Job drawing, mm, ordinate dimensions from the low corner. One solid piece. A direction names the side the tool comes from. Coordinates: 2 decimals unless noted, no trailing zeros. Write each loop counter-clockwise with the first axis right and the second up, starting at its lowest first coordinate (ties: lowest second). Pieces come first, ordered by that corner, then holes.
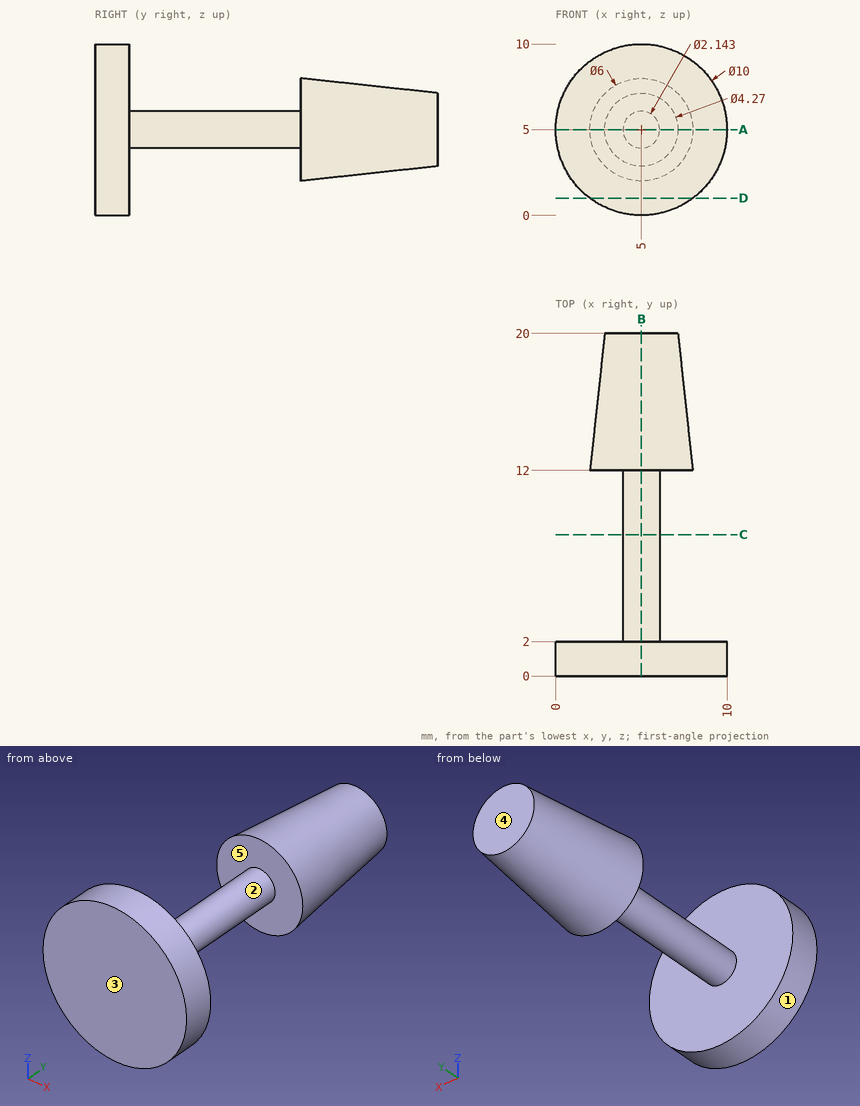
1. Saw through at C-C on y = 8.25. List the corners of the cut face in (x, z).
Computed values:
outline: circle Ø2.14 at (5, 5)
2. Saw through at A-A on z = 5. List the corners of the cut face in (x, y) (1 decimal).
Computed values:
outline: (0, 0) - (10, 0) - (10, 2) - (6.1, 2) - (6.1, 12) - (8, 12) - (7.1, 20) - (2.9, 20) - (2, 12) - (3.9, 12) - (3.9, 2) - (0, 2) - close
3. Saw through at B-B on x = 5. List the corners of the cut face in (y, z) (1 decimal).
Computed values:
outline: (0, 0) - (2, 0) - (2, 3.9) - (12, 3.9) - (12, 2) - (20, 2.9) - (20, 7.1) - (12, 8) - (12, 6.1) - (2, 6.1) - (2, 10) - (0, 10) - close
4. Flat gauge pins, fed straight in: pin 1 (6 mm diameter, centred on x = 3, y = 8.5, fed in from -Z); pin 2 (1.5 mm diameter, centred on x = 5.5, y = 16, fed in from +Z) (1 decimal); pin 3 (4 mm diameter, centred on x = 4.5, y = 10.5, fed in from -Z). Where does each tip first touch, or does it go through?
Computed values:
pin 1: stops at z = 3.93
pin 2: stops at z = 7.6
pin 3: stops at z = 2
5. Saw through at D-D on z = 1. List the corners of the cut face in (x, y).
Computed values:
outline: (2, 0) - (8, 0) - (8, 2) - (2, 2) - close
6. Mould opens along Y. For the marked faces 1, 2 and 3 say: +Y half, -Y half, draft (parallel to the pull), parting line (faces both ways), or undercut.
Computed values:
face 1: draft
face 2: undercut
face 3: -Y half
7. 3-axis set-ups, long thin cutter, end or side, ignore diameter. For the marked faces 4 and 5: which of +Z, -Z, +X, -X, +Y, -Y reach the whole face in a straight line?
Computed values:
face 4: +Z, -Z, +X, -X, +Y
face 5: none
8. Probe line 1 along Y through (x, z) = (6, 3.5); line 2 along Y through (x, z) = (8.25, 1.25); line 3 along Z through (x, y) = (5, 9.5). List the from-to ranges inside material, lowest first.
Computed values:
line 1: y = 0 to 2, 12 to 20
line 2: y = 0 to 2
line 3: z = 3.93 to 6.07
